from build123d import *

# Parameters (mm, degrees)
SKETCH2_R                            = 3.35
F_40_SERIES_TS40_40LM_650033_1_DEPTH = 250


with BuildPart() as part:
    # Sketch2 → 40 series TS40-40LM-650033(1) (new body)
    with BuildSketch(Plane(origin=(-125, 0, 0), x_dir=(0, 0, -1), z_dir=(1, 0, 0))):
        with BuildLine():
            Line((-7.7064, 0), (-7.7064, 5.551138531))
            Line((-7.7064, 5.551138531), (-13.331261469, 11.176))
            Line((-13.331261469, 11.176), (-16.6472, 11.176))
            Line((-16.6472, 11.176), (-16.6472, 7.6835))
            Line((-16.6472, 7.6835), (-15.2502, 7.6835))
            Line((-15.2502, 7.6835), (-15.2502, 4.0005))
            Line((-15.2502, 4.0005), (-20, 4.0005))
            Line((-20, 4.0005), (-20, 16.825))
            ThreePointArc((-20, 16.825), (-19.07006403, 19.07006403), (-16.825, 20))
            Line((-16.825, 20), (-4.0005, 20))
            Line((-4.0005, 20), (-4.0005, 15.2502))
            Line((-4.0005, 15.2502), (-7.6835, 15.2502))
            Line((-7.6835, 15.2502), (-7.6835, 16.6472))
            Line((-7.6835, 16.6472), (-11.176, 16.6472))
            Line((-11.176, 16.6472), (-11.176, 13.331261469))
            Line((-11.176, 13.331261469), (-5.551138531, 7.7064))
            Line((-5.551138531, 7.7064), (0, 7.7064))
            Line((0, 7.7064), (5.551138531, 7.7064))
            Line((5.551138531, 7.7064), (11.176, 13.331261469))
            Line((11.176, 13.331261469), (11.176, 16.6472))
            Line((11.176, 16.6472), (7.6835, 16.6472))
            Line((7.6835, 16.6472), (7.6835, 15.2502))
            Line((7.6835, 15.2502), (4.0005, 15.2502))
            Line((4.0005, 15.2502), (4.0005, 20))
            Line((4.0005, 20), (16.825, 20))
            ThreePointArc((16.825, 20), (19.07006403, 19.07006403), (20, 16.825))
            Line((20, 16.825), (20, 4.0005))
            Line((20, 4.0005), (15.2502, 4.0005))
            Line((15.2502, 4.0005), (15.2502, 7.6835))
            Line((15.2502, 7.6835), (16.6472, 7.6835))
            Line((16.6472, 7.6835), (16.6472, 11.176))
            Line((16.6472, 11.176), (13.331261469, 11.176))
            Line((13.331261469, 11.176), (7.7064, 5.551138531))
            Line((7.7064, 5.551138531), (7.7064, 0))
            Line((7.7064, 0), (7.7064, -5.551138531))
            Line((7.7064, -5.551138531), (13.331261469, -11.176))
            Line((13.331261469, -11.176), (16.6472, -11.176))
            Line((16.6472, -11.176), (16.6472, -7.6835))
            Line((16.6472, -7.6835), (15.2502, -7.6835))
            Line((15.2502, -7.6835), (15.2502, -4.0005))
            Line((15.2502, -4.0005), (20, -4.0005))
            Line((20, -4.0005), (20, -16.825))
            ThreePointArc((20, -16.825), (19.07006403, -19.07006403), (16.825, -20))
            Line((16.825, -20), (4.0005, -20))
            Line((4.0005, -20), (4.0005, -15.2502))
            Line((4.0005, -15.2502), (7.6835, -15.2502))
            Line((7.6835, -15.2502), (7.6835, -16.6472))
            Line((7.6835, -16.6472), (11.176, -16.6472))
            Line((11.176, -16.6472), (11.176, -13.331261469))
            Line((11.176, -13.331261469), (5.551138531, -7.7064))
            Line((5.551138531, -7.7064), (0, -7.7064))
            Line((0, -7.7064), (-5.551138531, -7.7064))
            Line((-5.551138531, -7.7064), (-11.176, -13.331261469))
            Line((-11.176, -13.331261469), (-11.176, -16.6472))
            Line((-11.176, -16.6472), (-7.6835, -16.6472))
            Line((-7.6835, -16.6472), (-7.6835, -15.2502))
            Line((-7.6835, -15.2502), (-4.0005, -15.2502))
            Line((-4.0005, -15.2502), (-4.0005, -20))
            Line((-4.0005, -20), (-16.825, -20))
            ThreePointArc((-16.825, -20), (-19.07006403, -19.07006403), (-20, -16.825))
            Line((-20, -16.825), (-20, -4.0005))
            Line((-20, -4.0005), (-15.2502, -4.0005))
            Line((-15.2502, -4.0005), (-15.2502, -7.6835))
            Line((-15.2502, -7.6835), (-16.6472, -7.6835))
            Line((-16.6472, -7.6835), (-16.6472, -11.176))
            Line((-16.6472, -11.176), (-13.331261469, -11.176))
            Line((-13.331261469, -11.176), (-7.7064, -5.551138531))
            Line((-7.7064, -5.551138531), (-7.7064, 0))
        make_face()
        Circle(SKETCH2_R, mode=Mode.SUBTRACT)
        with BuildLine():
            Line((18.222, 12.8372), (18.222, 15.428))
            ThreePointArc((18.222, 15.428), (17.403656347, 17.403656347), (15.428, 18.222))
            Line((15.428, 18.222), (12.8372, 18.222))
            Line((12.8372, 18.222), (12.8372, 12.8372))
            Line((12.8372, 12.8372), (18.222, 12.8372))
        make_face(mode=Mode.SUBTRACT)
        with BuildLine():
            Line((12.8372, -12.8372), (18.222, -12.8372))
            Line((18.222, -12.8372), (18.222, -15.428))
            ThreePointArc((18.222, -15.428), (17.403656347, -17.403656347), (15.428, -18.222))
            Line((15.428, -18.222), (12.8372, -18.222))
            Line((12.8372, -18.222), (12.8372, -12.8372))
        make_face(mode=Mode.SUBTRACT)
        with BuildLine():
            Line((-18.222, -12.8372), (-18.222, -15.428))
            ThreePointArc((-18.222, -15.428), (-17.403656347, -17.403656347), (-15.428, -18.222))
            Line((-15.428, -18.222), (-12.8372, -18.222))
            Line((-12.8372, -18.222), (-12.8372, -12.8372))
            Line((-12.8372, -12.8372), (-18.222, -12.8372))
        make_face(mode=Mode.SUBTRACT)
        with BuildLine():
            Line((-12.8372, 12.8372), (-18.222, 12.8372))
            Line((-18.222, 12.8372), (-18.222, 15.428))
            ThreePointArc((-18.222, 15.428), (-17.403656347, 17.403656347), (-15.428, 18.222))
            Line((-15.428, 18.222), (-12.8372, 18.222))
            Line((-12.8372, 18.222), (-12.8372, 12.8372))
        make_face(mode=Mode.SUBTRACT)
    extrude(amount=F_40_SERIES_TS40_40LM_650033_1_DEPTH)


solid = part.part
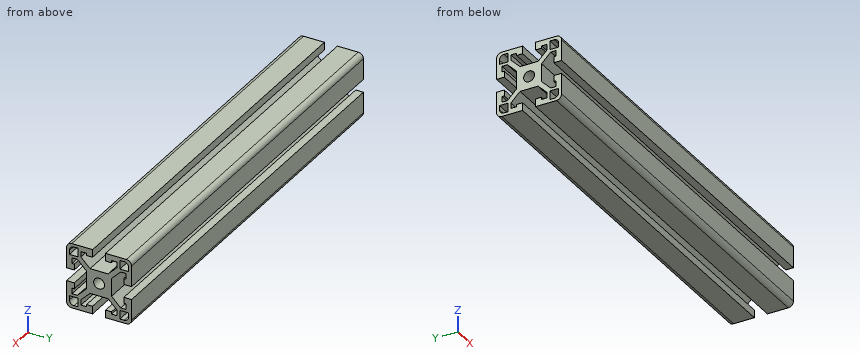
Source: CAD feature listing. Evaluate the final solid. Frame: model axes, mm. Coordinates: 2 decimals unless noted, no trailing zeros. Order: outer loops, then holes, each group sorted by start corner. A loop starts at its lowest first (then second) coordinate and runs counter-clockwise, first axis right, second up.
Item 1: First-contact query: P1, Ø1.5, axis at y = -13, z = 4.5, coming from the +X side; P2, Ø1, axis at x = 32.5, z = 0.5, coming from the +Y side. Flat tips, straight axial feed; report the tip coordinate or a pass-through.
Output values:
P1: passes through
P2: stops at y = 7.71
Item 2: Material intervals for line 1 (Y direction, x = -50, z = 13.5); line 2 (Z direction, x = 32.5, y = 15.5); line 3 (Y direction, x = -74, z = 0), sorted ascending.
Output values:
line 1: y = -20 to -18.22, -12.84 to -11.18, 11.18 to 12.84, 18.22 to 20
line 2: z = -20 to -18.22, -12.84 to -11.18, -7.68 to -4, 4 to 7.68, 11.18 to 12.84, 18.22 to 20
line 3: y = -7.71 to -3.35, 3.35 to 7.71
Item 3: Cut plane A-A (y = 0). Return loops of the section in (x, z).
Output values:
outline: (-125, -7.71) - (125, -7.71) - (125, -3.35) - (-125, -3.35) - close; (-125, 3.35) - (125, 3.35) - (125, 7.71) - (-125, 7.71) - close
Item 4: Cut plane C-C (x = -66). Count the separate pieces of the cut face and the enclosed holes in it, plus the area to 3 significant figures.
Output values:
separate pieces: 1
enclosed holes: 5
area: 708 mm2
